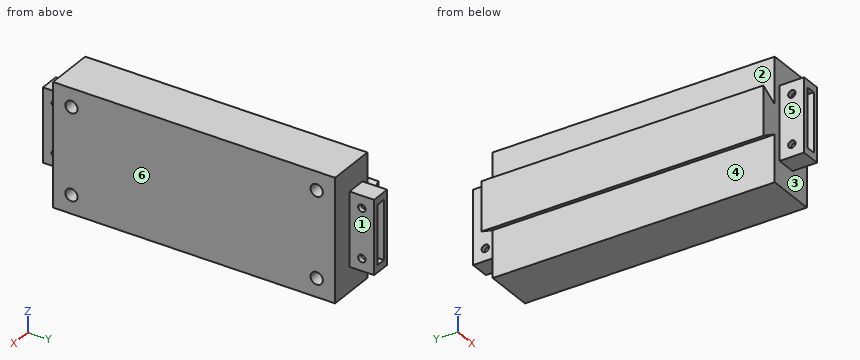
from build123d import *

# Parameters (mm, degrees)
BOSS_EXTRUDE1_DEPTH = 115
SKETCH2_R           = 2.5
CUT_EXTRUDE1_DEPTH  = 10
SKETCH3_W           = 8
SKETCH3_H           = 30
BOSS_EXTRUDE2_DEPTH = 10
SKETCH4_W           = 8
SKETCH4_H           = 30
BOSS_EXTRUDE3_DEPTH = 10
SKETCH5_W           = 4
SKETCH5_H           = 24
CUT_EXTRUDE2_DEPTH  = 10
SKETCH6_W           = 4
SKETCH6_H           = 24
CUT_EXTRUDE3_DEPTH  = 10
SKETCH7_R           = 1.5
CUT_EXTRUDE4_DEPTH  = 32


with BuildPart() as part:
    # Sketch1 → Boss-Extrude1 (new body)
    with BuildSketch(Plane(origin=(0, 0, 0), x_dir=(1, 0, 0), z_dir=(0, 1, 0))):
        Polygon((-27, 10), (-27, -10), (-20, -5.958548116), (-20, -25), (0, -25), (0, 25), (-20, 25), (-20, 5.958548116), align=None)
    extrude(amount=BOSS_EXTRUDE1_DEPTH)

    # Sketch2 → Cut-Extrude1 (cut)
    with BuildSketch(Plane(origin=(0, 0, 0), x_dir=(0, 0, -1), z_dir=(1, 0, 0))):
        with Locations((-17.5, 107.5)):
            Circle(SKETCH2_R)
        with Locations((-17.5, 7.5)):
            Circle(SKETCH2_R)
        with Locations((17.5, 7.5)):
            Circle(SKETCH2_R)
        with Locations((17.5, 107.5)):
            Circle(SKETCH2_R)
    extrude(amount=-CUT_EXTRUDE1_DEPTH, mode=Mode.SUBTRACT)

    # Sketch3 → Boss-Extrude2 (add)
    with BuildSketch(Plane(origin=(0, 115, 0), x_dir=(1, 0, 0), z_dir=(0, 1, 0))):
        with Locations((-13, 0)):
            Rectangle(SKETCH3_W, SKETCH3_H)
    extrude(amount=BOSS_EXTRUDE2_DEPTH)

    # Sketch4 → Boss-Extrude3 (add)
    with BuildSketch(Plane.XZ):
        with Locations((-13, 0)):
            Rectangle(SKETCH4_W, SKETCH4_H)
    extrude(amount=BOSS_EXTRUDE3_DEPTH)

    # Sketch5 → Cut-Extrude2 (cut)
    with BuildSketch(Plane.XZ.offset(10)):
        with Locations((-13, 0)):
            Rectangle(SKETCH5_W, SKETCH5_H)
    extrude(amount=-CUT_EXTRUDE2_DEPTH, mode=Mode.SUBTRACT)

    # Sketch6 → Cut-Extrude3 (cut)
    with BuildSketch(Plane(origin=(0, 125, 0), x_dir=(1, 0, 0), z_dir=(0, 1, 0))):
        with Locations((-13, 0)):
            Rectangle(SKETCH6_W, SKETCH6_H)
    extrude(amount=-CUT_EXTRUDE3_DEPTH, mode=Mode.SUBTRACT)

    # Sketch7 → Cut-Extrude4 (cut)
    with BuildSketch(Plane(origin=(0, 0, 0), x_dir=(0, 0, -1), z_dir=(1, 0, 0))):
        with Locations((-10, 120)):
            Circle(SKETCH7_R)
        with Locations((-10, -5)):
            Circle(SKETCH7_R)
        with Locations((10, -5)):
            Circle(SKETCH7_R)
        with Locations((10, 120)):
            Circle(SKETCH7_R)
    extrude(amount=-CUT_EXTRUDE4_DEPTH, mode=Mode.SUBTRACT)


solid = part.part
Could you check a few things on this model? Use its own coordinates, in mm. Face numbers are marked on the shaded views. A direction names the side the tool comes from. Round coordinates to 2 decimals unless told otherwise and drop trailing zeros. Loops run counter-clockwise (first coordinate to the right, second up) from the corner with the lowest first, then second, coordinate; pieces in that order, holes last. Notation, with made-up numbers: (-0.75, 23) - (22.25, 23) arc R27 cw to (22.25, 42) - close; hole circle Ø8 at (86.5, 77.25). An arc over 180 degrees is marked (long way). Write item = value, one per line.
1) Imagine slicing it at B-B (x = -13). Please give me the cut outline in (y, z).
Computed:
outline = (-10, -15) - (0, -15) - (0, -25) - (115, -25) - (115, -15) - (125, -15) - (125, -12) - (115, -12) - (115, 12) - (125, 12) - (125, 15) - (115, 15) - (115, 25) - (0, 25) - (0, 15) - (-10, 15) - (-10, 12) - (0, 12) - (0, -12) - (-10, -12) - close
2) I'm going to push flat-ended pins straight in: P1, Ø4, axis at x = -21.5, z = -7.5, coming from the -Y side; P2, Ø2.5, axis at y = 120, z = 10, coming from the -X side; P3, Ø3.5, axis at y = -5, z = -10, coming from the +X side; P4, Ø3, axis at y = 7.5, z = -17.5, coming from the +X side. Where does each tip first touch, or does it pass through?
Computed:
P1 = 0
P2 = through
P3 = -9
P4 = -10
3) Imagine slicing it at A-A (y = -5). Please give me the cut outline in (x, z).
Computed:
outline = (-17, -15) - (-9, -15) - (-9, -11.5) - (-11, -11.5) - (-11, -12) - (-15, -12) - (-15, -11.5) - (-17, -11.5) - close; (-17, -8.5) - (-15, -8.5) - (-15, 8.5) - (-17, 8.5) - close; (-17, 11.5) - (-15, 11.5) - (-15, 12) - (-11, 12) - (-11, 11.5) - (-9, 11.5) - (-9, 15) - (-17, 15) - close; (-11, -8.5) - (-9, -8.5) - (-9, 8.5) - (-11, 8.5) - close
4) Imagine slicing it at D-D (x = -3). Please give me the cut outline in (y, z).
Computed:
outline = (0, -25) - (115, -25) - (115, 25) - (0, 25) - close; hole circle Ø5 at (7.5, -17.5); hole circle Ø5 at (7.5, 17.5); hole circle Ø5 at (107.5, -17.5); hole circle Ø5 at (107.5, 17.5)
5) I need wall thicknesses on line 1 along Y through (x, z) = (-9.45, -10); line 2 along Z through (x, y) = (-15.65, 120); line 3 along X through (y, z) = (119.5, 1.5). Which ranges of each line are inside material? Lowest first, please. Write a range as from..to.
Computed:
line_1 = -10..-6.5, -3.5..118.5, 121.5..125
line_2 = -15..-11.5, -8.5..8.5, 11.5..15
line_3 = -17..-15, -11..-9
6) On a 3-axis mill with a long thin cutter (end or side, diameter ignored), from which of +Z, -Z, +X, -X, +Y, -Y can I reach the whole of each face in a straight line? I mean the marked faces 4, 5 and 6. Say none if no direction works.
Computed:
face_4 = -Z, +Y, -Y
face_5 = +Z, -Z, -X, -Y
face_6 = +Z, -Z, +X, +Y, -Y
7) Imagine slicing it at C-C (z = 17.5). Please give me the cut outline in (x, y), and give its area (3 significant figures).
Computed:
outline = (-20, 0) - (0, 0) - (0, 5) - (-10, 5) - (-10, 10) - (0, 10) - (0, 105) - (-10, 105) - (-10, 110) - (0, 110) - (0, 115) - (-20, 115) - close
area = 2,200 mm2
8) If we mould it in two halves opening along X, with no side actions, what happens to the marked faces 1, 2 and 3? For each: pulls with the +X half, pulls with the -X half, needs draft (parallel to the pull), parting line crosses it, or undercut.
Computed:
face_1 = pulls with the +X half
face_2 = undercut
face_3 = needs draft
